Autodesk Inventor part; units mm, degrees
ref_plane "YZ Plane" through (0, 0, 0) normal (1, 0, 0) x (0, 1, 0)
ref_plane "XZ Plane" through (0, 0, 0) normal (0, 1, 0) x (-1, 0, 0)
ref_plane "XY Plane" through (0, 0, 0) normal (0, 0, 1) x (1, 0, 0)
sketch "스케치1" plane through (0, 0, 0) normal (0, 0, 1) x (1, 0, 0)
  line L0 (-18, -16) -> (-18, 16)
  line L1 (-18, 16) -> (18, 16)
  line L2 (18, 16) -> (18, -16)
  line L3 (18, -16) -> (-18, -16)
  circle A0 centre (36.125, 36.075) radius 2.5
  circle A1 centre (-36.125, -36.075) radius 2.5
  circle A2 centre (36.075, -36.125) radius 2.5
  circle A3 centre (-36.075, 36.125) radius 2.5
  arc A4 (-39.6581, -32.537) -> (-32.5919, -39.613) centre (-36.125, -36.075) ccw
  line L4 (-32.5919, -39.613) -> (-17.9206, -24.962)
  arc A5 (-14.3876, -23.5) -> (-17.9206, -24.962) centre (-14.3876, -28.5) ccw
  line L5 (-14.3876, -23.5) -> (14.3282, -23.5)
  arc A6 (17.8662, -24.9669) -> (14.3282, -23.5) centre (14.3282, -28.5) ccw
  line L6 (17.8662, -24.9669) -> (32.537, -39.6581)
  arc A7 (32.537, -39.6581) -> (39.613, -32.5919) centre (36.075, -36.125) ccw
  line L7 (39.613, -32.5919) -> (24.962, -17.9206)
  arc A8 (23.5, -14.3876) -> (24.962, -17.9206) centre (28.5, -14.3876) ccw
  line L8 (23.5, -14.3876) -> (23.5, 14.3282)
  arc A9 (24.9669, 17.8662) -> (23.5, 14.3282) centre (28.5, 14.3282) ccw
  line L9 (24.9669, 17.8662) -> (39.6581, 32.537)
  arc A10 (39.6581, 32.537) -> (32.5919, 39.613) centre (36.125, 36.075) ccw
  line L10 (32.5919, 39.613) -> (17.9206, 24.962)
  arc A11 (14.3876, 23.5) -> (17.9206, 24.962) centre (14.3876, 28.5) ccw
  line L11 (14.3876, 23.5) -> (-14.3282, 23.5)
  arc A12 (-17.8662, 24.9669) -> (-14.3282, 23.5) centre (-14.3282, 28.5) ccw
  line L12 (-17.8662, 24.9669) -> (-32.537, 39.6581)
  arc A13 (-32.537, 39.6581) -> (-39.613, 32.5919) centre (-36.075, 36.125) ccw
  line L13 (-39.613, 32.5919) -> (-24.962, 17.9206)
  arc A14 (-23.5, 14.3876) -> (-24.962, 17.9206) centre (-28.5, 14.3876) ccw
  line L14 (-23.5, 14.3876) -> (-23.5, -14.3282)
  arc A15 (-24.9669, -17.8662) -> (-23.5, -14.3282) centre (-28.5, -14.3282) ccw
  line L15 (-24.9669, -17.8662) -> (-39.6581, -32.537)
  circle A16 centre (0, 0) radius 65
  dimension "d38" = 72.2
  dimension "d39" = 72.2
  dimension "d62" = 130
extrude "돌출3" add sketch "스케치1" along normal blind 4 contours L0 L1 L2 L3 | A0 | A1 | A2 | A3 | L15 A15 L14 A14 L13 A13 L12 A12 L11 A11 L10 A10 L9 A9 L8 A8 L7 A7 L6 A6 L5 A5 L4 A4 | A16
sketch "스케치6" plane through (0, 0, 4) normal (0, 0, 1) x (1, 0, 0)
  line L0 (0, 0) -> (60.0652, -60.0652) construction
  line L1 (0, 0) -> (84.945, 0) construction
  circle A0 centre (42.4264, -42.4264) radius 1.5
  circle A1 centre (0, 0) radius 60 construction
  circle A2 centre (0, 0) radius 60 construction
  circle A3 centre (60, 0) radius 1.5
  circle A4 centre (0, 0) radius 60 construction
  circle A5 centre (42.4264, 42.4264) radius 1.5
  circle A6 centre (0, 0) radius 60 construction
  circle A7 centre (0, 60) radius 1.5
  circle A8 centre (0, 0) radius 60 construction
  circle A9 centre (-42.4264, 42.4264) radius 1.5
  circle A10 centre (0, 0) radius 60 construction
  circle A11 centre (-60, 0) radius 1.5
  circle A12 centre (0, 0) radius 60 construction
  circle A13 centre (-42.4264, -42.4264) radius 1.5
  circle A14 centre (0, 0) radius 60 construction
  circle A15 centre (0, -60) radius 1.5
  circle A16 centre (0, 0) radius 65
  dimension "d65" = 120
  dimension "d63" = 45
  dimension "d64" = 3
  dimension "d68" = 360
  dimension "d72" = 130
extrude "돌출4" cut sketch "스케치6" against normal through all contours A0 | A3 | A5 | A7 | A9 | A11 | A13 | A15
sketch "스케치7" plane through (0, 0, 4) normal (0, 0, 1) x (1, 0, 0)
  circle A0 centre (-36.075, 36.125) radius 2.5
  circle A1 centre (36.075, -36.125) radius 2.5
  circle A2 centre (-36.125, -36.075) radius 2.5
  circle A3 centre (36.125, 36.075) radius 2.5
  circle A4 centre (-42.4264, -42.4264) radius 1.5
  circle A5 centre (-42.4264, 42.4264) radius 1.5
  circle A6 centre (42.4264, 42.4264) radius 1.5
  circle A7 centre (42.4264, -42.4264) radius 1.5
  circle A8 centre (60, 0) radius 1.5
  circle A9 centre (0, 60) radius 1.5
  circle A10 centre (-60, 0) radius 1.5
  circle A11 centre (0, -60) radius 1.5
  circle A12 centre (-42.4264, -42.4264) radius 1.5
  circle A13 centre (-42.4264, 42.4264) radius 1.5
  circle A14 centre (42.4264, 42.4264) radius 1.5
  circle A15 centre (42.4264, -42.4264) radius 1.5
  circle A16 centre (60, 0) radius 1.5
  circle A17 centre (0, 60) radius 1.5
  circle A18 centre (-60, 0) radius 1.5
  circle A19 centre (0, -60) radius 1.5
  circle A20 centre (0, 0) radius 65
  circle A21 centre (-36.075, 36.125) radius 2.5
  circle A22 centre (36.125, 36.075) radius 2.5
  circle A23 centre (-36.125, -36.075) radius 2.5
  circle A24 centre (36.075, -36.125) radius 2.5
  circle A25 centre (-47.1805, -19.5045) radius 2.5
  circle A26 centre (19.5045, -47.1805) radius 2.5
  circle A27 centre (47.1805, 19.5045) radius 2.5
  circle A28 centre (-19.5045, 47.1805) radius 2.5
  dimension "d76" = 67.5
extrude "돌출5" cut sketch "스케치7" against normal through all contours A25 | A26 | A27 | A28
sketch "스케치8" plane through (0, 0, 4) normal (0, 0, 1) x (1, 0, 0)
  circle A0 centre (-19.5045, 47.1805) radius 2.5
  circle A1 centre (0, 0) radius 65
  circle A2 centre (0, 0) radius 24.5 construction
  line L0 (0, 0) -> (-19.5045, 47.1805) construction
  point P0 (-9.3601, 22.6415)
  dimension "d80" = 49
hole "구멍5" at (-9.3601, 22.6415, 4) direction (0, 0, -1) diameter 2.459 end through all
pattern_circular "원형 패턴1" count 4 over 360 about axis through (0, 0, 0) along (0, 0, 1) of "구멍5"
sketch "스케치9" plane through (0, 0, 0) normal (0, 0, -1) x (-1, 0, 0)
  circle A0 centre (42.4264, 42.4264) radius 1.5
  circle A1 centre (0, 60) radius 1.5
  circle A2 centre (-42.4264, 42.4264) radius 1.5
  circle A3 centre (-60, 0) radius 1.5
  circle A4 centre (-42.4264, -42.4264) radius 1.5
  circle A5 centre (0, -60) radius 1.5
  circle A6 centre (42.4264, -42.4264) radius 1.5
  circle A7 centre (60, 0) radius 1.5
  circle A8 centre (18.5456, 40.1536) radius 1.5
  circle A9 centre (-41.5066, 15.2792) radius 1.5
  circle A10 centre (41.5066, -15.2792) radius 1.5
  circle A11 centre (-18.5456, -40.1536) radius 1.5
  circle A12 centre (0, 0) radius 65
  line L0 (-4.3465, 36.6246) -> (-6.6426, 42.1678)
  line L1 (-9.2557, 43.2502) -> (-24.0378, 37.1273)
  line L2 (-25.1202, 34.5142) -> (-22.8241, 28.9709)
  arc A13 (-37.7646, 20.6175) -> (-38.847, 18.0044) centre (-36.9993, 18.7698) ccw
  line L3 (-38.847, 18.0044) -> (-37.699, 15.2327)
  arc A14 (-38.7814, 12.6196) -> (-37.699, 15.2327) centre (-39.5467, 14.4674) ccw
  line L4 (-38.7814, 12.6196) -> (-41.553, 11.4716)
  arc A15 (-41.553, 11.4716) -> (-42.6354, 8.8584) centre (-40.7876, 9.6238) ccw
  line L5 (-42.6354, 8.8584) -> (-23.8839, -36.4117)
  arc A16 (-23.8839, -36.4117) -> (-21.2708, -37.494) centre (-22.0362, -35.6463) ccw
  line L6 (-21.2708, -37.494) -> (-18.4992, -36.346)
  arc A17 (-15.886, -37.4284) -> (-18.4992, -36.346) centre (-17.7338, -38.1938) ccw
  line L7 (-15.886, -37.4284) -> (-14.738, -40.2)
  arc A18 (-14.738, -40.2) -> (-12.1249, -41.2824) centre (-12.8902, -39.4347) ccw
  line L8 (-12.1249, -41.2824) -> (37.7646, -20.6175)
  arc A19 (37.7646, -20.6175) -> (38.847, -18.0044) centre (36.9993, -18.7698) ccw
  line L9 (38.847, -18.0044) -> (37.699, -15.2327)
  arc A20 (38.7814, -12.6196) -> (37.699, -15.2327) centre (39.5467, -14.4674) ccw
  line L10 (38.7814, -12.6196) -> (41.553, -11.4716)
  arc A21 (41.553, -11.4716) -> (42.6354, -8.8584) centre (40.7876, -9.6238) ccw
  line L11 (42.6354, -8.8584) -> (23.8839, 36.4117)
  arc A22 (23.8839, 36.4117) -> (21.2708, 37.494) centre (22.0362, 35.6463) ccw
  line L12 (21.2708, 37.494) -> (18.4992, 36.346)
  arc A23 (15.886, 37.4284) -> (18.4992, 36.346) centre (17.7338, 38.1938) ccw
  line L13 (15.886, 37.4284) -> (14.738, 40.2)
  arc A24 (14.738, 40.2) -> (12.1249, 41.2824) centre (12.8902, 39.4347) ccw
  line L14 (12.1249, 41.2824) -> (-1.7333, 35.5422)
  line L15 (-7.4079, 44.0156) -> (-25.8789, 36.346)
  line L16 (-25.8789, 36.346) -> (-22.0507, 27.1264)
  line L17 (-7.4079, 44.0156) -> (-3.5797, 34.796)
  line L18 (-3.5797, 34.796) -> (-22.0507, 27.1264)
extrude "돌출6" cut sketch "스케치9" against normal through all contours L17 L18 L16 L15
fillet "모깎기1" radius 2 4 edges at (25.8789, 36.346, 2) (22.0507, 27.1264, 2) (3.5797, 34.796, 2) (7.4079, 44.0156, 2)
sketch "스케치10" plane through (0, 0, 4) normal (0, 0, 1) x (1, 0, 0)
  line L0 (25.112, 34.4989) -> (22.8177, 28.9735)
  arc A0 (20.2036, 27.8934) -> (22.8177, 28.9735) centre (20.9706, 29.7405) ccw
  line L1 (20.2036, 27.8934) -> (5.4268, 34.0291)
  arc A1 (4.3467, 36.6431) -> (5.4268, 34.0291) centre (6.1938, 35.8762) ccw
  line L2 (4.3467, 36.6431) -> (6.641, 42.1685)
  arc A2 (9.255, 43.2486) -> (6.641, 42.1685) centre (8.4881, 41.4015) ccw
  line L3 (9.255, 43.2486) -> (24.0318, 37.113)
  arc A3 (25.112, 34.4989) -> (24.0318, 37.113) centre (23.2649, 35.2659) ccw
  circle A4 centre (22.6415, 9.3601) radius 1.2295
  circle A5 centre (9.3601, -22.6415) radius 1.2295
  circle A6 centre (-22.6415, -9.3601) radius 1.2295
  circle A7 centre (-9.3601, 22.6415) radius 1.2295
  circle A8 centre (47.1805, 19.5045) radius 2.5
  circle A9 centre (-47.1805, -19.5045) radius 2.5
  circle A10 centre (19.5045, -47.1805) radius 2.5
  circle A11 centre (-19.5045, 47.1805) radius 2.5
  circle A12 centre (-42.4264, -42.4264) radius 1.5
  circle A13 centre (-42.4264, 42.4264) radius 1.5
  circle A14 centre (42.4264, 42.4264) radius 1.5
  circle A15 centre (42.4264, -42.4264) radius 1.5
  circle A16 centre (60, 0) radius 1.5
  circle A17 centre (0, 60) radius 1.5
  circle A18 centre (-60, 0) radius 1.5
  circle A19 centre (0, -60) radius 1.5
  circle A20 centre (0, 0) radius 65
  circle A21 centre (0, 0) radius 29
  line L4 (0, 0) -> (59.5002, 0) construction
  circle A22 centre (18.9196, 15.5659) radius 1
  line L5 (18.9196, 15.5659) -> (0, 0)
  circle A23 centre (0, 0) radius 24.5 construction
  dimension "d96" = 2
extrude "돌출7" cut sketch "스케치10" against normal through all contours A22
properties part number "CPU면 철판가공"
Work out the finished part from the listing and answer in its coordinate system (mm). A direction names the side the tool comes from. Give positions to 0.01 mm unless a question says otherwise; leave off trailing zeros. Write each loop counter-clockwise with the first axis right and the second up, starting at its lowest first coordinate (ties: lowest second). Pieces come first, ordered by that corner, then holes. Notation, with made-up numbers: (7, 28.25) - (57, 28.25) arc R28 ccw to (57, 54.25) - close; hole circle Ø7 at (30, -30.75). An arc over 180 degrees is marked (long way). One line per item, written item: value. Start each with the question number.
1. Consider probe 1 along Y at (x, z) = (0, 0.95); probe 2 along Y at (x, z) = (-43, 1.6); probe 3 along X at (y, z) = (18.5, 3.6). Determine where each line is inside the solid, lowest interval first.
2. For a pull along X with two mould halves and no side action, classify faces 1 (the flat face through (-1, 1, 0)), 2 (the cylindrical face through (62, -19.52, 1.97)), 3 (the cylindrical face through (41.236, -43.339, 2.028)) as +X half, -X half, draft (parallel to the pull), parting line (faces both ways), or undercut.
3. Given pin 1 (2 mm diameter, centred on y = 2, z = 3, fed in from -X); pin 2 (2 mm diameter, centred on y = -14, z = 1.5, fed in from -X); pin 3 (2 mm diameter, centred on y = 12, z = 3, fed in from +X), each flat-ended and moving along its own axis, determine where each tip first touches the part or whether it passes through.
4. Find section B-B (x = 0). Write down the section's boundary in (y, z), then the cut area to 3 significant figures.
5. Find section A-A (x = 60). Write down the section's boundary in (y, z).
6. For faces 4 (the flat face through (-1, 1, 4)), 5 (the flat face through (5.51, 39.44, 1.97)), determine the directions among +Z, -Z, +X, -X, +Y, -Y from which every point of the face is accessible in a straight line to the end or side of a thin tool.
Geometry results:
1. probe 1: -65 to -61.5, -58.5 to 58.5, 61.5 to 65
1. probe 2: -48.74 to -43.81, -41.04 to 41.04, 43.81 to 48.74
1. probe 3: -62.31 to 44.89, 49.47 to 62.31
2. face 1: draft
2. face 2: parting line
2. face 3: undercut
3. pin 1: x = -64.99
3. pin 2: x = -63.69
3. pin 3: x = 64.06
4. outline: (-65, 0) - (-61.5, 0) - (-61.5, 4) - (-65, 4) - close; (-58.5, 0) - (58.5, 0) - (58.5, 4) - (-58.5, 4) - close; (61.5, 0) - (65, 0) - (65, 4) - (61.5, 4) - close
4. area: 496 mm2
5. outline: (-25, 0) - (-1.5, 0) - (-1.5, 4) - (-25, 4) - close; (1.5, 0) - (25, 0) - (25, 4) - (1.5, 4) - close
6. face 4: +Z, +X, -X, +Y, -Y
6. face 5: +Z, -Z
